Geometry check sheet. Reference: the model listing, model coordinates, mm. Face numbers are marked on the shaded views. A direction names the side the tool comes from. Round coordinates to 2 decimals unless told otherwise and drop trailing zeros. Loops run counter-clockwise (first coordinate to the right, second up) from the corner with the lowest first, then second, coordinate; pieces in that order, holes last. Notation, with made-up numbers: (45, 39.25) -> (96, 39.25) arc R31 ccw to (96, 76.25) -> close; hole circle Ø3 at (13.5, 86). An arc over 180 degrees is marked (long way). Use one line per item in the form item = value.
from build123d import *

# Parameters (mm, degrees)
ESQUISSE2_R        = 6
BOSS_EXTRU_1_DEPTH = 15


with BuildPart() as part:
    # Esquisse1 → Révolution1 (revolve)
    with BuildSketch(Plane.XY):
        Polygon((0, 0), (45, 0), (45, -27), (50, -27), (50, -22), (47, -22), (47, -17), (50, -17), (50, -14), (47, -14), (47, -9), (50, -9), (50, -6), (57.5, -6), (57.5, 6), (0, 6), align=None)
    revolve(axis=Axis((0, 0, 0), (0, 1, 0)))

    # Esquisse2 → Boss.-Extru.1 (add)
    with BuildSketch(Plane(origin=(0, 6, 0), x_dir=(1, 0, 0), z_dir=(0, 1, 0))):
        with Locations(Location((0, 30, 0), (0, 0, 180))):
            Circle(ESQUISSE2_R)
        with Locations(Location((28.531695489, 9.270509831, 0), (0, 0, 180))):
            Circle(ESQUISSE2_R)
        with Locations(Location((17.633557569, -24.270509831, 0), (0, 0, 180))):
            Circle(ESQUISSE2_R)
        with Locations(Location((-17.633557569, -24.270509831, 0), (0, 0, 180))):
            Circle(ESQUISSE2_R)
        with Locations(Location((-28.531695489, 9.270509831, 0), (0, 0, 180))):
            Circle(ESQUISSE2_R)
    extrude(amount=BOSS_EXTRU_1_DEPTH)


solid = part.part
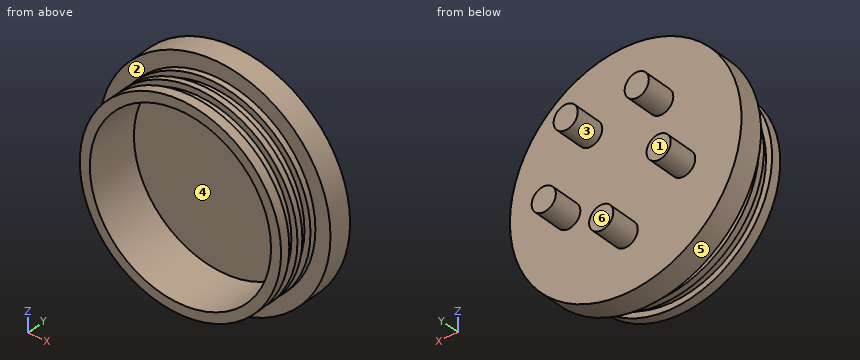
1. Section check B-B (z = 0). Record the boundary of the cut face in (x, y).
Return value:
outline = (-57.5, -6) -> (-50, -6) -> (-50, -9) -> (-47, -9) -> (-47, -14) -> (-50, -14) -> (-50, -17) -> (-47, -17) -> (-47, -22) -> (-50, -22) -> (-50, -27) -> (-45, -27) -> (-45, 0) -> (45, 0) -> (45, -27) -> (50, -27) -> (50, -22) -> (47, -22) -> (47, -17) -> (50, -17) -> (50, -14) -> (47, -14) -> (47, -9) -> (50, -9) -> (50, -6) -> (57.5, -6) -> (57.5, 6) -> (-57.5, 6) -> close
2. Gauge pin test, flat ends, axial feed: pin 1 (3 mm diameter, centred on x = -25.5, z = -1.5, fed in from +Y); pin 2 (4 mm diameter, centred on y = -6, z = 5, fed in from -X); pin 3 (1 mm diameter, centred on x = 8.5, y = -20.5, fed in from +Z). Record the tip position at first contact, or that the pin passes through.
Return value:
pin_1 = 6
pin_2 = -57.42
pin_3 = 46.31
3. Mould release check, pull along Z, two halves, no side actions. Record for the marked faces 4, 5 and 6: released by +Z, released by -Z, zero draft, split by the parting line, or undercut.
Return value:
face_4 = undercut
face_5 = split by the parting line
face_6 = zero draft
4. Material ranges on line 1 along Y through (x, z) = (9, 48); line 2 along X through (y, z) = (-7, 0), recorded low to high.
Return value:
line_1 = -27 to -22, -17 to -14, -9 to 6
line_2 = -50 to -45, 45 to 50
5. Section check C-C (y = 14.5). Record the boundary of the cut face in (x, z), then the cut area to 3 significant figures.
Return value:
outline = circle Ø12 at (-28.53, -9.27); circle Ø12 at (-17.63, 24.27); circle Ø12 at (0, -30); circle Ø12 at (17.63, 24.27); circle Ø12 at (28.53, -9.27)
area = 565 mm2
6. Tool access check on the marked faces 1, 2 and 3. Record the directions out of +Z, -Z, +X, -X, +Y, -Y that give a thin tool (end or side, any length) a straight path to the whole face; none if there is none.
Return value:
face_1 = +Z, -Z, +X, -X, +Y
face_2 = -Y
face_3 = +Y
7. Section check D-D (y = 4). Record the boundary of the cut face in (x, z), then the cut area to 3 significant figures.
Return value:
outline = circle Ø115 at (0, 0)
area = 10,400 mm2
